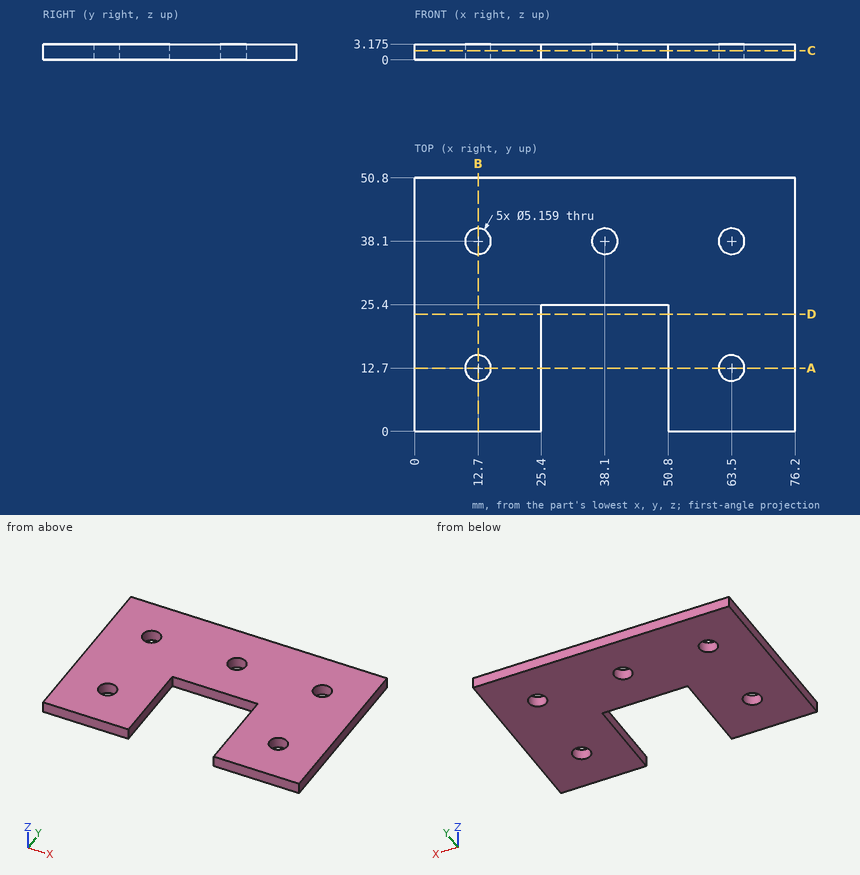
The drawing under review shows one solid part. Ordinate dimensions are in mm from its lowest x, y, z. Coordinates: 2 decimals unless noted, no trailing zeros. Write each loop counter-clockwise with the first axis right and the second up, starting at its lowest first coordinate (ties: lowest second). Pieces come first, ordered by that corner, then holes.
1) Add section B-B (x = 12.7). Write out the cut boundary in (y, z) (1 decimal).
2) To check wall thickness, follow L1, parallel to Y at x = 12.7, z = 1.5; L2, parallel to Y at x = 38.1, z = 1; L3, parallel to X at y = 7.5, z = 1.75. State the ranges of each line that lie inside material, in increasing order.
3) Add section C-C (z = 1.85). Write out the cut boundary in (x, y).
4) Add section A-A (y = 12.7). Write out the cut boundary in (x, z) (1 decimal).
5) Insertion check: pin 1 (4 mm diameter, centred on x = 63.5, y = 12.7, fed in from -Z); pin 2 (1.6 mm diameter, centred on y = 17.5, z = 2.5, fed in from -X); pin 3 (1 mm diameter, centred on x = 40, z = 1.5, fed in from -Y). Each pin has a flat end and moves straight along its axis. Give the tip position at first contact, or say it passes through.
6) Add section D-D (y = 23.5). Write out the cut boundary in (x, z) (1 decimal).
Check result:
1. outline: (0, 0) - (10.1, 0) - (10.1, 3.2) - (0, 3.2) - close; (15.3, 0) - (35.5, 0) - (35.5, 3.2) - (15.3, 3.2) - close; (40.7, 0) - (50.8, 0) - (50.8, 3.2) - (40.7, 3.2) - close
2. L1: y = 0 to 10.12, 15.28 to 35.52, 40.68 to 50.8
2. L2: y = 25.4 to 35.52, 40.68 to 50.8
2. L3: x = 0 to 25.4, 50.8 to 76.2
3. outline: (0, 0) - (25.4, 0) - (25.4, 25.4) - (50.8, 25.4) - (50.8, 0) - (76.2, 0) - (76.2, 50.8) - (0, 50.8) - close; hole circle Ø5.16 at (12.7, 12.7); hole circle Ø5.16 at (12.7, 38.1); hole circle Ø5.16 at (38.1, 38.1); hole circle Ø5.16 at (63.5, 12.7); hole circle Ø5.16 at (63.5, 38.1)
4. outline: (0, 0) - (10.1, 0) - (10.1, 3.2) - (0, 3.2) - close; (15.3, 0) - (25.4, 0) - (25.4, 3.2) - (15.3, 3.2) - close; (50.8, 0) - (60.9, 0) - (60.9, 3.2) - (50.8, 3.2) - close; (66.1, 0) - (76.2, 0) - (76.2, 3.2) - (66.1, 3.2) - close
5. pin 1: passes through
5. pin 2: stops at x = 0
5. pin 3: stops at y = 25.4
6. outline: (0, 0) - (25.4, 0) - (25.4, 3.2) - (0, 3.2) - close; (50.8, 0) - (76.2, 0) - (76.2, 3.2) - (50.8, 3.2) - close
